```python
from build123d import *

# Parameters (mm, degrees)
PAD_DEPTH           = 10
SKETCH001_R         = 2.75
SKETCH001_R_2       = 1.8
POCKET_DEPTH        = 15.001
POCKET001_DEPTH     = 3
SKETCH003_R         = 5.1
POCKET002_DEPTH     = 2
SKETCH004_R         = 1.9
PAD001_DEPTH        = 0.2
SKETCH005_R         = 2.95
PAD002_DEPTH        = 0.2
PAD003_DEPTH        = 0.2
LINEARPATTERN_COUNT = 6
LINEARPATTERN_PITCH = 3.96
POCKET003_DEPTH     = 2
CHAMFER_SIZE        = 5
CHAMFER001_SIZE     = 0.8


with BuildPart() as part:
    # Sketch → Pad (new body, symmetric)
    with BuildSketch(Plane.XZ):
        with BuildLine():
            ThreePointArc((3.976179, 8.9), (-4.068927, 7.396182), (4.1, 7.9))
            Line((4.1, 7.9), (8.5, 7.9))
            Line((8.5, 7.9), (10, 6.4))
            Line((10, 6.4), (10, 5))
            Line((10, 5), (22, 5))
            Line((22, 5), (22, 0))
            Line((-20, 0), (22, 0))
            Line((-20, 0), (-20, 5))
            Line((-20, 5), (-8, 5))
            Line((-8, 5), (-8, 10))
            ThreePointArc((-3, 15), (-6.535534, 13.535534), (-8, 10))
            Line((-3, 15), (10, 15))
            Line((10, 15), (10, 10.4))
            Line((8.5, 8.9), (10, 10.4))
            Line((8.5, 8.9), (3.976179, 8.9))
        make_face()
    extrude(amount=PAD_DEPTH, both=True)

    # Sketch001 → Pocket (cut, through all)
    with BuildSketch(Plane(origin=(0, 0, 0), x_dir=(1, 0, 0), z_dir=(0, 0, -1))):
        with Locations((-14, 0)):
            Circle(SKETCH001_R)
        with Locations((16, 0)):
            Circle(SKETCH001_R)
        with Locations((6.5, 0)):
            Circle(SKETCH001_R_2)
    extrude(amount=-POCKET_DEPTH, mode=Mode.SUBTRACT)

    # Sketch002 → Pocket001 (cut)
    with BuildSketch(Plane(origin=(0, 0, 0), x_dir=(1, 0, 0), z_dir=(0, 0, -1))):
        Polygon((6.5, 3.406367), (3.55, 1.703183), (3.55, -1.703183), (6.5, -3.406367), (9.45, -1.703183), (9.45, 1.703183), align=None)
    extrude(amount=-POCKET001_DEPTH, mode=Mode.SUBTRACT)

    # Sketch003 → Pocket002 (cut)
    with BuildSketch(Plane.XY.offset(5)):
        with Locations((-14, 0)):
            Circle(SKETCH003_R)
        with Locations((16, 0)):
            Circle(SKETCH003_R)
    extrude(amount=-POCKET002_DEPTH, mode=Mode.SUBTRACT)

    # Sketch004 → Pad001 (join)
    with BuildSketch(Plane.XY.offset(8.9)):
        with Locations((6.5, 0)):
            Circle(SKETCH004_R)
    extrude(amount=PAD001_DEPTH)

    # Sketch005 → Pad002 (join)
    with BuildSketch(Plane.XY.offset(3)):
        with Locations((6.5, 0)):
            Circle(SKETCH005_R)
    extrude(amount=PAD002_DEPTH)

    # Sketch006 → Pad003 (join)
    with BuildSketch(Plane.XZ.offset(-10)):
        with BuildLine():
            ThreePointArc((4.1, 7.9), (4.068927, 8.403818), (3.976179, 8.9))
            Line((8.5, 8.9), (3.976179, 8.9))
            Line((8.5, 7.9), (8.5, 8.9))
            Line((4.1, 7.9), (8.5, 7.9))
        make_face()
    pad003 = extrude(amount=PAD003_DEPTH)

    # LinearPattern: Pad003 ×6
    with Locations(*[(0, -i * LINEARPATTERN_PITCH, 0) for i in range(1, LINEARPATTERN_COUNT)]):
        add(pad003)

    # Sketch007 → Pocket003 (cut)
    with BuildSketch(Plane.XY.offset(15)):
        with BuildLine():
            ThreePointArc((6.5, 3.65), (2.85, 0), (6.5, -3.65))
            Line((10.5, -3.65), (6.5, -3.65))
            Line((10.5, 3.65), (10.5, -3.65))
            Line((6.5, 3.65), (10.5, 3.65))
        make_face()
    extrude(amount=-POCKET003_DEPTH, mode=Mode.SUBTRACT)

    # Chamfer
    chamfer_edges = [part.edges().sort_by_distance(p)[0] for p in [
        (22, -10, 2.5),
        (-20, -10, 2.5),
        (22, 10, 2.5),
        (-20, 10, 2.5),
    ]]
    chamfer(chamfer_edges, length=CHAMFER_SIZE)

    # Chamfer001
    chamfer001_edges = [part.edges().sort_by_distance(p)[0] for p in [
        (-8, -10, 7.5),
        (-6.535534, -10, 13.535534),
        (3.5, -10, 15),
        (3.5, 10, 15),
        (-6.535534, 10, 13.535534),
        (-8, 10, 7.5),
    ]]
    chamfer(chamfer001_edges, length=CHAMFER001_SIZE)


solid = part.part
```
Can you work these out from the model? Positions are in its coordinate system, mm. A direction names the side the tool comes from. Coordinates: 2 decimals unless noted, no trailing zeros. Loops run counter-clockwise (first coordinate to the right, second up) from the corner with the lowest first, then second, coordinate; pieces in that order, holes last. Notation, with made-up numbers: M -21,-1.75 L 15,-1.75 A19 cw 15,27.25 Z; hole C -40,-37 d9. An arc over 180 degrees is marked long. Put each result on its own line as item: value. Start each with the question number.
(1) Imagine slicing it at A-A on x = 16. List the corners of the cut face in (y, z) for me.
(2) Will these pins go through, and if not, where does the flat tip stop? pin 1 Ø5 at (y, z) = (2, 9.5) entering from -X; pin 2 Ø6 at (x, y) = (16, -0.5) entering from +Z; pin 3 Ø1.8 at (x, y) = (6.5, 0) entering from +Z.
(3) Imagine slicing it at C-C on y = -6.75. List the corners of the cut face in (x, z) for me, and give its area (3 significant figures).
(4) We'd pull the mould along Y, two halves only. Please class faces 1 (the face through (-6.09, 9.87, 13.03)), 2 (the face through (8.217, -0.541, 5.517)), 3 (the face through (22, 0, 3)): +Y half, -Y half, draft (parallel to the pull), parting line (faces both ways), or undercut.
(5) Imagine slicing it at B-B on z = 1. List the corners of the cut face in (x, y) for me.
(6) I need wall thicknesses on probe 1 along Z at (x, y) = (0, -5.5); probe 2 along X at (y, z) = (0, 1.8); probe 3 along Y at (x, z) = (7, 8.25). Which ranges of each line are inside material? Lowest first, please.
(7) Which directions (+Z, -Z, +X, -X, +Y, -Y) give clear straight access to the entire face, cutting with the end or side of a thin tool? Please do faces 4 (the face through (3.55, 0, 1)), 5 (the face through (-11.8, -2.2, 3)), 6 (the face through (6, 8, 8.9)).
(8) Imagine slicing it at D-D on x = 11.5. List the corners of the cut face in (y, z) for me.
Worked answers:
1. outline: M -10,0 L -2.75,0 L -2.75,3 L -5.1,3 L -5.1,5 L -10,5 Z; M 2.75,0 L 10,0 L 10,5 L 5.1,5 L 5.1,3 L 2.75,3 Z
2. pin 1: stops at x = -8
2. pin 2: stops at z = 3
2. pin 3: stops at z = 9.1
3. outline: M -18.25,0 L 20.25,0 L 20.25,5 L 10,5 L 10,6.4 L 8.5,7.9 L 4.1,7.9 A4.1 cw long 3.98,8.9 L 8.5,8.9 L 10,10.4 L 10,15 L -3,15 A5 ccw -8,10 L -8,5 L -18.25,5 Z
3. area: 306 mm2
4. face 1: +Y half
4. face 2: undercut
4. face 3: draft
5. outline: M -20,-5 L -15,-10 L 17,-10 L 22,-5 L 22,5 L 17,10 L -15,10 L -20,5 Z; hole C -14,0 d5.5; hole M 3.55,-1.7 L 6.5,-3.41 L 9.45,-1.7 L 9.45,1.7 L 6.5,3.41 L 3.55,1.7 Z; hole C 16,0 d5.5
6. probe 1: z = 0 to 3.8, 12 to 15
6. probe 2: x = -20 to -16.75, -11.25 to 3.55, 9.45 to 13.25, 18.75 to 22
6. probe 3: y = -10 to -9.8, -6.04 to -5.84, -2.08 to -1.88, 1.88 to 2.08, 5.84 to 6.04, 9.8 to 10
7. face 4: -Z
7. face 5: +Z
7. face 6: +X
8. outline: M -10,0 L 10,0 L 10,5 L 2.4,5 L 2.4,3 L -2.4,3 L -2.4,5 L -10,5 Z
